```python
from build123d import *

# Parameters (mm, degrees)
BOSS_EXTRUDE1_DEPTH = 5
SKETCH2_R           = 2.125
CUT_EXTRUDE1_DEPTH  = 3
SKETCH4_R           = 2.6
SKETCH4_R_2         = 1.6
CUT_EXTRUDE3_DEPTH  = 10
SKETCH5_R           = 2.1
CUT_EXTRUDE4_DEPTH  = 10
FILLET1_R           = 10
SKETCH6_R           = 2.6
CUT_EXTRUDE5_DEPTH  = 10


with BuildPart() as part:
    # Sketch1 → Boss-Extrude1 (new body)
    with BuildSketch(Plane(origin=(0, 0, 0), x_dir=(1, 0, 0), z_dir=(0, 1, 0))):
        Polygon((130, 352), (-130, 352), (-130, 110), (-380, 110), (-380, -110), (-130, -110), (-130, -352), (130, -352), (130, -110), (380, -110), (380, 110), (130, 110), align=None)
    extrude(amount=BOSS_EXTRUDE1_DEPTH)

    # Sketch2 → Cut-Extrude1 (cut)
    with BuildSketch(Plane(origin=(0, 5, 0), x_dir=(1, 0, 0), z_dir=(0, 1, 0))):
        with Locations(Location((330, 49.5, 0), (0, 0, 270))):
            Circle(SKETCH2_R)
        with Locations(Location((305, 49.5, 0), (0, 0, 270))):
            Circle(SKETCH2_R)
        with Locations(Location((327.5, 19.5, 0), (0, 0, 270))):
            Circle(SKETCH2_R)
        with Locations(Location((327.5, -19.5, 0), (0, 0, 90))):
            Circle(SKETCH2_R)
        with Locations(Location((305, -49.5, 0), (0, 0, 90))):
            Circle(SKETCH2_R)
        with Locations(Location((330, -49.5, 0), (0, 0, 90))):
            Circle(SKETCH2_R)
        with Locations(Location((-330, -49.5, 0), (0, 0, 270))):
            Circle(SKETCH2_R)
        with Locations(Location((-305, -49.5, 0), (0, 0, 270))):
            Circle(SKETCH2_R)
        with Locations(Location((-327.5, -19.5, 0), (0, 0, 270))):
            Circle(SKETCH2_R)
        with Locations(Location((-327.5, 19.5, 0), (0, 0, 90))):
            Circle(SKETCH2_R)
        with Locations(Location((-305, 49.5, 0), (0, 0, 90))):
            Circle(SKETCH2_R)
        with Locations(Location((-330, 49.5, 0), (0, 0, 90))):
            Circle(SKETCH2_R)
        with Locations(Location((47.5, 302, 0), (0, 0, 270))):
            Circle(SKETCH2_R)
        with Locations(Location((47.5, 277, 0), (0, 0, 270))):
            Circle(SKETCH2_R)
        with Locations(Location((-47.5, 277, 0), (0, 0, 90))):
            Circle(SKETCH2_R)
        with Locations(Location((-47.5, 302, 0), (0, 0, 90))):
            Circle(SKETCH2_R)
        with Locations(Location((-47.5, -302, 0), (0, 0, 270))):
            Circle(SKETCH2_R)
        with Locations(Location((-47.5, -277, 0), (0, 0, 270))):
            Circle(SKETCH2_R)
        with Locations(Location((47.5, -277, 0), (0, 0, 90))):
            Circle(SKETCH2_R)
        with Locations(Location((47.5, -302, 0), (0, 0, 90))):
            Circle(SKETCH2_R)
    extrude(amount=-CUT_EXTRUDE1_DEPTH, mode=Mode.SUBTRACT)

    # Sketch4 → Cut-Extrude3 (cut)
    with BuildSketch(Plane(origin=(0, 5, 0), x_dir=(1, 0, 0), z_dir=(0, 1, 0))):
        with Locations(Location((-122, 192, 0), (0, 0, 270))):
            Circle(SKETCH4_R)
        with Locations(Location((-110, 192, 0), (0, 0, 270))):
            Circle(SKETCH4_R)
        with Locations(Location((-122, 217, 0), (0, 0, 270))):
            Circle(SKETCH4_R)
        with Locations(Location((-122, 237, 0), (0, 0, 270))):
            Circle(SKETCH4_R)
        with Locations(Location((-122, 262, 0), (0, 0, 270))):
            Circle(SKETCH4_R)
        with Locations(Location((-110, 262, 0), (0, 0, 270))):
            Circle(SKETCH4_R)
        with Locations(Location((110, 262, 0), (0, 0, 90))):
            Circle(SKETCH4_R)
        with Locations(Location((122, 262, 0), (0, 0, 90))):
            Circle(SKETCH4_R)
        with Locations(Location((122, 237, 0), (0, 0, 90))):
            Circle(SKETCH4_R)
        with Locations(Location((122, 217, 0), (0, 0, 90))):
            Circle(SKETCH4_R)
        with Locations(Location((110, 192, 0), (0, 0, 90))):
            Circle(SKETCH4_R)
        with Locations(Location((122, 192, 0), (0, 0, 90))):
            Circle(SKETCH4_R)
        with Locations(Location((122, -192, 0), (0, 0, 270))):
            Circle(SKETCH4_R)
        with Locations(Location((110, -192, 0), (0, 0, 270))):
            Circle(SKETCH4_R)
        with Locations(Location((122, -217, 0), (0, 0, 270))):
            Circle(SKETCH4_R)
        with Locations(Location((122, -237, 0), (0, 0, 270))):
            Circle(SKETCH4_R)
        with Locations(Location((122, -262, 0), (0, 0, 270))):
            Circle(SKETCH4_R)
        with Locations(Location((110, -262, 0), (0, 0, 270))):
            Circle(SKETCH4_R)
        with Locations(Location((-110, -262, 0), (0, 0, 90))):
            Circle(SKETCH4_R)
        with Locations(Location((-122, -262, 0), (0, 0, 90))):
            Circle(SKETCH4_R)
        with Locations(Location((-122, -237, 0), (0, 0, 90))):
            Circle(SKETCH4_R)
        with Locations(Location((-122, -217, 0), (0, 0, 90))):
            Circle(SKETCH4_R)
        with Locations(Location((-110, -192, 0), (0, 0, 90))):
            Circle(SKETCH4_R)
        with Locations(Location((-122, -192, 0), (0, 0, 90))):
            Circle(SKETCH4_R)
        with Locations(Location((109, -227, 0), (0, 0, 270))):
            Circle(SKETCH4_R_2)
        with Locations(Location((-109, -227, 0), (0, 0, 90))):
            Circle(SKETCH4_R_2)
        with Locations(Location((109, 227, 0), (0, 0, 90))):
            Circle(SKETCH4_R_2)
        with Locations(Location((-109, 227, 0), (0, 0, 270))):
            Circle(SKETCH4_R_2)
        with Locations(Location((99, -227, 0), (0, 0, 270))):
            Circle(SKETCH4_R_2)
        with Locations(Location((-99, -227, 0), (0, 0, 90))):
            Circle(SKETCH4_R_2)
        with Locations(Location((99, 227, 0), (0, 0, 90))):
            Circle(SKETCH4_R_2)
        with Locations(Location((-99, 227, 0), (0, 0, 270))):
            Circle(SKETCH4_R_2)
    extrude(amount=-CUT_EXTRUDE3_DEPTH, mode=Mode.SUBTRACT)

    # Sketch5 → Cut-Extrude4 (cut)
    with BuildSketch(Plane(origin=(0, 5, 0), x_dir=(1, 0, 0), z_dir=(0, 1, 0))):
        with Locations(Location((-50, 347, 0), (0, 0, 270))):
            Circle(SKETCH5_R)
        with Locations(Location((50, 347, 0), (0, 0, 270))):
            Circle(SKETCH5_R)
        with Locations(Location((50, -347, 0), (0, 0, 90))):
            Circle(SKETCH5_R)
        with Locations(Location((-50, -347, 0), (0, 0, 90))):
            Circle(SKETCH5_R)
        with Locations(Location((-375, 50, 0), (0, 0, 270))):
            Circle(SKETCH5_R)
        with Locations(Location((-375, -50, 0), (0, 0, 270))):
            Circle(SKETCH5_R)
        with Locations(Location((375, -50, 0), (0, 0, 90))):
            Circle(SKETCH5_R)
        with Locations(Location((375, 50, 0), (0, 0, 90))):
            Circle(SKETCH5_R)
    extrude(amount=-CUT_EXTRUDE4_DEPTH, mode=Mode.SUBTRACT)

    # Fillet1
    fillet1_edges = [part.edges().sort_by_distance(p)[0] for p in [
        (130, 2.5, -110),
        (130, 2.5, 110),
        (-130, 2.5, 110),
        (-130, 2.5, -110),
    ]]
    fillet(fillet1_edges, radius=FILLET1_R)

    # Sketch6 → Cut-Extrude5 (cut)
    with BuildSketch(Plane(origin=(0, 5, 0), x_dir=(1, 0, 0), z_dir=(0, 1, 0))):
        with Locations(Location((-110, 312, 0), (0, 0, 270))):
            Circle(SKETCH6_R)
        with Locations(Location((-68.4, 312, 0), (0, 0, 270))):
            Circle(SKETCH6_R)
        with Locations(Location((68.4, 312, 0), (0, 0, 90))):
            Circle(SKETCH6_R)
        with Locations(Location((110, 312, 0), (0, 0, 90))):
            Circle(SKETCH6_R)
        with Locations(Location((110, -312, 0), (0, 0, 270))):
            Circle(SKETCH6_R)
        with Locations(Location((68.4, -312, 0), (0, 0, 270))):
            Circle(SKETCH6_R)
        with Locations(Location((-68.4, -312, 0), (0, 0, 90))):
            Circle(SKETCH6_R)
        with Locations(Location((-110, -312, 0), (0, 0, 90))):
            Circle(SKETCH6_R)
        with Locations(Location((258.4, 80, 0), (0, 0, 270))):
            Circle(SKETCH6_R)
        with Locations(Location((300, 80, 0), (0, 0, 270))):
            Circle(SKETCH6_R)
        with Locations(Location((300, -80, 0), (0, 0, 90))):
            Circle(SKETCH6_R)
        with Locations(Location((258.4, -80, 0), (0, 0, 90))):
            Circle(SKETCH6_R)
        with Locations(Location((-258.4, -80, 0), (0, 0, 270))):
            Circle(SKETCH6_R)
        with Locations(Location((-300, -80, 0), (0, 0, 270))):
            Circle(SKETCH6_R)
        with Locations(Location((-300, 80, 0), (0, 0, 90))):
            Circle(SKETCH6_R)
        with Locations(Location((-258.4, 80, 0), (0, 0, 90))):
            Circle(SKETCH6_R)
    extrude(amount=-CUT_EXTRUDE5_DEPTH, mode=Mode.SUBTRACT)


solid = part.part
```
The listing builds one solid part. Answer for the finished solid, in the listing's coordinates (mm). Round coordinates to 2 decimals unless told otherwise and drop trailing zeros. Order: outer loops, then holes, each group sorted by start corner. A loop starts at its lowest first (then second) coordinate and runs counter-clockwise, first axis right, second up. Notation, with made-up numbers: (23, 26) - (57, 26) arc R26 ccw to (57, 43) - close; hole circle Ø6 at (81.25, 79). An arc over 180 degrees is marked (long way). Put each result on its own line as item: value. Start each with the question number.
(1) Given P1, Ø1.3, axis at x = -47, z = -301.5, coming from the +Y side; P2, Ø7, axis at x = -122, z = 192, coming from the +Y side; P3, Ø1.5, axis at y = 3.5, z = 186, coming from the +X side; P4, Ø3, axis at x = -300, z = 80, coming from the +Y side, each flat-ended and moving along its own axis, determine where each tip first touches the part or whether it passes through.
(2) Find section A-A (y = 2.9). State how many separate pieces and enclosed holes the cut face has, plus the area to 3 significant figures.
(3) Straight lines are drawn through the part: probe 1 along X at (y, z) = (3.9, -227); probe 2 along X at (y, z) = (3.25, 80); probe 3 along Z at (x, y) = (327.5, 3) (3 decimals). For each, find the intervals that lie inside material, in ascending order. Write a range as from..to.
(4) Find section B-B (z = 167). Give the vertices of the cut face in (x, y), plus the area to 3 significant figures.
(5) Find section C-C (x = 247). Give the vertices of the cut face in (y, z).
Reply:
1. P1: y = 2
1. P2: y = 5
1. P3: x = 130
1. P4: through
2. separate pieces: 1
2. enclosed holes: 76
2. area: 292,000 mm^2
3. probe 1: -130..-110.6, -107.4..-100.6, -97.4..97.4, 100.6..107.4, 110.6..130
3. probe 2: -380..-302.6, -297.4..-261, -255.8..255.8, 261..297.4, 302.6..380
3. probe 3: -110..-21.625, -17.375..17.375, 21.625..110
4. outline: (-130, 0) - (130, 0) - (130, 5) - (-130, 5) - close
4. area: 1,300 mm^2
5. outline: (0, -110) - (5, -110) - (5, 110) - (0, 110) - close
